from build123d import *

# Parameters (mm, degrees)
ESQUISSE1_R          = 8
ESQUISSE1_R_2        = 3
BASE_EXTRUSION_DEPTH = 2


with BuildPart() as part:
    # Esquisse1 → Base-Extrusion (new, symmetric)
    with BuildSketch(Plane.XY):
        with BuildLine():
            Line((1.064516129, 11.9526903), (62.576612903, 6.474373913))
            ThreePointArc((62.576612903, 6.474373913), (68.5, 0), (62.576612903, -6.474373913))
            Line((62.576612903, -6.474373913), (1.064516129, -11.9526903))
            ThreePointArc((1.064516129, -11.9526903), (-12, 0), (1.064516129, 11.9526903))
        make_face()
        Circle(ESQUISSE1_R, mode=Mode.SUBTRACT)
        with Locations((62, 0)):
            Circle(ESQUISSE1_R_2, mode=Mode.SUBTRACT)
        with BuildLine():
            Line((14.266129032, 6.76111181), (53.266129032, 3.287740712))
            ThreePointArc((53.266129032, 3.287740712), (55.213412196, 2.324612939), (56, 0.299568137))
            Line((56, 0.299568137), (56, -0.299568137))
            ThreePointArc((56, -0.299568137), (55.213412196, -2.324612939), (53.266129032, -3.287740712))
            Line((53.266129032, -3.287740712), (14.266129032, -6.76111181))
            ThreePointArc((14.266129032, -6.76111181), (11.974955198, -5.98635143), (11, -3.772939235))
            Line((11, -3.772939235), (11, 3.772939235))
            ThreePointArc((11, 3.772939235), (11.974955198, 5.98635143), (14.266129032, 6.76111181))
        make_face(mode=Mode.SUBTRACT)
    extrude(amount=BASE_EXTRUSION_DEPTH, both=True)


solid = part.part
Input: part model. Units: mm. Frame: model coordinates. A direction names the side the tool comes from. Coordinates: 2 decimals unless noted, no trailing zeros. Order: outer loops, then holes, each group sorted by start corner. A loop starts at its lowest first (then second) coordinate and runs counter-clockwise, first axis right, second up.
1. Draft query along Y for faces 1 (the cylindrical face through (12, -6.01, 0.03)), 2 (the flat face through (31.39, 9.25, 0.03)), 3 (the flat face through (33.49, 5.05, 0.03)), 4 (the cylindrical face through (-12, 0, 0)). Return one class per face: +Y half, -Y half, draft (parallel to the pull), parting line (faces both ways), or undercut.
Checked values:
face 1: undercut
face 2: +Y half
face 3: undercut
face 4: parting line
2. Cut plane B-B, the plane y = -5.5. Return loops of the section in (x, z), plus the area to 3 significant figures.
Checked values:
outline: (-10.67, -2) - (-5.81, -2) - (-5.81, 2) - (-10.67, 2) - close; (5.81, -2) - (11.55, -2) - (11.55, 2) - (5.81, 2) - close; (28.43, -2) - (65.46, -2) - (65.46, 2) - (28.43, 2) - close
area: 191 mm2
3. Ray query, line 1 along X through (y, z) = (2.5, -0.45); line 2 along Y through (x, z) = (42, 1.3); line 3 along Y through (x, z) = (47, 1.35). Return the intervals inside material, ascending.
Checked values:
line 1: x = -11.74 to -7.6, 7.6 to 11, 55.04 to 60.34, 63.66 to 68
line 2: y = -8.31 to -4.29, 4.29 to 8.31
line 3: y = -7.86 to -3.85, 3.85 to 7.86
4. Cut plane D-D, the plane x = 41. Return loops of the section in (y, z).
Checked values:
outline: (-8.4, -2) - (-4.38, -2) - (-4.38, 2) - (-8.4, 2) - close; (4.38, -2) - (8.4, -2) - (8.4, 2) - (4.38, 2) - close
5. Cut plane A-A, the plane x = 0. Return loops of the section in (y, z).
Checked values:
outline: (-12, -2) - (-8, -2) - (-8, 2) - (-12, 2) - close; (8, -2) - (12, -2) - (12, 2) - (8, 2) - close
6. Access query for faces 5 (the flat face through (29, 6, -2)), 6 (the flat face through (11, 0, 0)). Directions: +Z, -Z, +X, -X, +Y, -Y. A direction counts if a zero-diameter tool reaches every point of the face in a straight line with its end or side. Return the directions, or none.
Checked values:
face 5: -Z, +X, -X, +Y, -Y
face 6: +Z, -Z
7. Cut plane C-C, the plane z = -0.45. Return loops of the section in (x, y), plus the area to 3 significant figures.
Checked values:
outline: (1.06, -11.95) - (62.58, -6.47) arc R6.5 ccw to (62.58, 6.47) - (1.06, 11.95) arc R12 ccw (long way) to start; hole circle Ø16 at (0, 0); hole (11, -3.77) arc R3 ccw to (14.27, -6.76) - (53.27, -3.29) arc R3 ccw to (56, -0.3) - (56, 0.3) arc R3 ccw to (53.27, 3.29) - (14.27, 6.76) arc R3 ccw to (11, 3.77) - close; hole circle Ø6 at (62, 0)
area: 768 mm2
8. Contact query for flat-ended pins moving along their axis: P1, Ø2, axis at x = 15, z = 0.5, coming from the +Y side; P2, Ø2, axis at x = 41.5, z = 1, coming from the -Y side; P3, Ø2, axis at y = 6.5, z = -1, coming from the +X side. Output: stop coordinate, or through.
Checked values:
P1: stops at y = 10.8
P2: stops at y = -8.44
P3: stops at x = 65.46
